Geometry check sheet. Reference: the model listing, model coordinates, mm. Give positions to 0.01 mm unless a question says otherwise; leave off trailing zeros. Loops run counter-clockwise (first coordinate to the right, second up) from the corner with the lowest first, then second, coordinate; pieces in that order, holes last. Notation, with made-up numbers: (85, 27.5) -> (132, 27.5) arc R19 cw to (132, 46.5) -> close; hole circle Ø2 at (48, 84.5). An arc over 180 degrees is marked (long way). One line per item, written item: value. Start each with the question number.
(1) Scan lines: line 1 along Y through (x, z) = (19, 1.2) (3 decimals); line 2 along Y through (x, z) = (-104.5, 1.9) (3 decimals); line 3 along Y through (x, z) = (24, 0.5) (3 decimals). Record each from-to range of solid material in increasing order. Write a range as from..to.
(2) Sectioned sample at C-C, the plane z = 0.55. State how many separate pieces and enclosed holes the cut face has, then the cut area to 3 significant figures.
(3) Sectioned sample at A-A, the plane x = 95.25. Record the cut outline in (y, z) (3 decimals).
(4) Draft check along X on faces 1 (the face through (-2, -3, 0)), 2 (the face through (103.9, 0.95, 1.57)). Enter one of: pulls with the +X half, pulls with the -X half, needs draft (parallel to the pull), parting line crosses it, or undercut.
(5) Sectioned sample at B-B, the plane x = -76.2. Record the cut outline in (y, z) (3 decimals).
Autodesk Inventor part; units mm, degrees
ref_plane "YZ Plane" through (0, 0, 0) normal (1, 0, 0) x (0, 1, 0)
ref_plane "XZ Plane" through (0, 0, 0) normal (0, 1, 0) x (-1, 0, 0)
ref_plane "XY Plane" through (0, 0, 0) normal (0, 0, 1) x (1, 0, 0)
sketch "Sketch1" plane through (0, 0, 0) normal (0, 0, 1) x (1, 0, 0)
  line L0 (-114.3, -15.875) -> (114.3, -15.875)
  line L1 (114.3, -15.875) -> (114.3, 15.875)
  line L2 (114.3, 15.875) -> (-114.3, 15.875)
  line L3 (-114.3, 15.875) -> (-114.3, -15.875)
  line L4 (-114.3, -15.875) -> (114.3, 15.875) construction
  line L5 (114.3, -15.875) -> (-114.3, 15.875) construction
  line L6 (-107.95, 9.525) -> (-82.55, 9.525) construction
  line L7 (-107.95, 6.9596) -> (-82.55, 6.9596)
  line L8 (-82.55, 12.0904) -> (-107.95, 12.0904)
  arc A0 (-107.95, 12.0904) -> (-107.95, 6.9596) centre (-107.95, 9.525) ccw
  arc A1 (-82.55, 6.9596) -> (-82.55, 12.0904) centre (-82.55, 9.525) ccw
  line L9 (-69.85, 9.525) -> (-44.45, 9.525) construction
  line L10 (-69.85, 6.9596) -> (-44.45, 6.9596)
  line L11 (-44.45, 12.0904) -> (-69.85, 12.0904)
  arc A2 (-69.85, 12.0904) -> (-69.85, 6.9596) centre (-69.85, 9.525) ccw
  arc A3 (-44.45, 6.9596) -> (-44.45, 12.0904) centre (-44.45, 9.525) ccw
  line L12 (-31.75, 9.525) -> (-6.35, 9.525) construction
  line L13 (-31.75, 6.9596) -> (-6.35, 6.9596)
  line L14 (-6.35, 12.0904) -> (-31.75, 12.0904)
  arc A4 (-31.75, 12.0904) -> (-31.75, 6.9596) centre (-31.75, 9.525) ccw
  arc A5 (-6.35, 6.9596) -> (-6.35, 12.0904) centre (-6.35, 9.525) ccw
  line L15 (6.35, 9.525) -> (31.75, 9.525) construction
  line L16 (6.35, 6.9596) -> (31.75, 6.9596)
  line L17 (31.75, 12.0904) -> (6.35, 12.0904)
  arc A6 (6.35, 12.0904) -> (6.35, 6.9596) centre (6.35, 9.525) ccw
  arc A7 (31.75, 6.9596) -> (31.75, 12.0904) centre (31.75, 9.525) ccw
  line L18 (44.45, 9.525) -> (69.85, 9.525) construction
  line L19 (44.45, 6.9596) -> (69.85, 6.9596)
  line L20 (69.85, 12.0904) -> (44.45, 12.0904)
  arc A8 (44.45, 12.0904) -> (44.45, 6.9596) centre (44.45, 9.525) ccw
  arc A9 (69.85, 6.9596) -> (69.85, 12.0904) centre (69.85, 9.525) ccw
  line L21 (82.55, 9.525) -> (107.95, 9.525) construction
  line L22 (82.55, 6.9596) -> (107.95, 6.9596)
  line L23 (107.95, 12.0904) -> (82.55, 12.0904)
  arc A10 (82.55, 12.0904) -> (82.55, 6.9596) centre (82.55, 9.525) ccw
  arc A11 (107.95, 6.9596) -> (107.95, 12.0904) centre (107.95, 9.525) ccw
  line L24 (-107.95, -9.525) -> (-82.55, -9.525) construction
  line L25 (-107.95, -12.0904) -> (-82.55, -12.0904)
  line L26 (-82.55, -6.9596) -> (-107.95, -6.9596)
  arc A12 (-107.95, -6.9596) -> (-107.95, -12.0904) centre (-107.95, -9.525) ccw
  arc A13 (-82.55, -12.0904) -> (-82.55, -6.9596) centre (-82.55, -9.525) ccw
  line L27 (-69.85, -9.525) -> (-44.45, -9.525) construction
  line L28 (-69.85, -12.0904) -> (-44.45, -12.0904)
  line L29 (-44.45, -6.9596) -> (-69.85, -6.9596)
  arc A14 (-69.85, -6.9596) -> (-69.85, -12.0904) centre (-69.85, -9.525) ccw
  arc A15 (-44.45, -12.0904) -> (-44.45, -6.9596) centre (-44.45, -9.525) ccw
  line L30 (-31.75, -9.525) -> (-6.35, -9.525) construction
  line L31 (-31.75, -12.0904) -> (-6.35, -12.0904)
  line L32 (-6.35, -6.9596) -> (-31.75, -6.9596)
  arc A16 (-31.75, -6.9596) -> (-31.75, -12.0904) centre (-31.75, -9.525) ccw
  arc A17 (-6.35, -12.0904) -> (-6.35, -6.9596) centre (-6.35, -9.525) ccw
  line L33 (6.35, -9.525) -> (31.75, -9.525) construction
  line L34 (6.35, -12.0904) -> (31.75, -12.0904)
  line L35 (31.75, -6.9596) -> (6.35, -6.9596)
  arc A18 (6.35, -6.9596) -> (6.35, -12.0904) centre (6.35, -9.525) ccw
  arc A19 (31.75, -12.0904) -> (31.75, -6.9596) centre (31.75, -9.525) ccw
  line L36 (44.45, -9.525) -> (69.85, -9.525) construction
  line L37 (44.45, -12.0904) -> (69.85, -12.0904)
  line L38 (69.85, -6.9596) -> (44.45, -6.9596)
  arc A20 (44.45, -6.9596) -> (44.45, -12.0904) centre (44.45, -9.525) ccw
  arc A21 (69.85, -12.0904) -> (69.85, -6.9596) centre (69.85, -9.525) ccw
  line L39 (82.55, -9.525) -> (107.95, -9.525) construction
  line L40 (82.55, -12.0904) -> (107.95, -12.0904)
  line L41 (107.95, -6.9596) -> (82.55, -6.9596)
  arc A22 (82.55, -6.9596) -> (82.55, -12.0904) centre (82.55, -9.525) ccw
  arc A23 (107.95, -12.0904) -> (107.95, -6.9596) centre (107.95, -9.525) ccw
  circle A24 centre (-107.95, 0) radius 2.4892
  circle A25 centre (-101.6, 0) radius 2.4892
  circle A26 centre (-95.25, 0) radius 2.4892
  circle A27 centre (-88.9, 0) radius 2.4892
  circle A28 centre (-82.55, 0) radius 2.4892
  circle A29 centre (-76.2, 0) radius 2.4892
  circle A30 centre (-69.85, 0) radius 2.4892
  circle A31 centre (-63.5, 0) radius 2.4892
  circle A32 centre (-57.15, 0) radius 2.4892
  circle A33 centre (-50.8, 0) radius 2.4892
  circle A34 centre (-44.45, 0) radius 2.4892
  circle A35 centre (-38.1, 0) radius 2.4892
  circle A36 centre (-31.75, 0) radius 2.4892
  circle A37 centre (-25.4, 0) radius 2.4892
  circle A38 centre (-19.05, 0) radius 2.4892
  circle A39 centre (-12.7, 0) radius 2.4892
  circle A40 centre (-6.35, 0) radius 2.4892
  circle A41 centre (0, 0) radius 2.4892
  circle A42 centre (6.35, 0) radius 2.4892
  circle A43 centre (12.7, 0) radius 2.4892
  circle A44 centre (19.05, 0) radius 2.4892
  circle A45 centre (25.4, 0) radius 2.4892
  circle A46 centre (31.75, 0) radius 2.4892
  circle A47 centre (38.1, 0) radius 2.4892
  circle A48 centre (44.45, 0) radius 2.4892
  circle A49 centre (50.8, 0) radius 2.4892
  circle A50 centre (57.15, 0) radius 2.4892
  circle A51 centre (63.5, 0) radius 2.4892
  circle A52 centre (69.85, 0) radius 2.4892
  circle A53 centre (76.2, 0) radius 2.4892
  circle A54 centre (82.55, 0) radius 2.4892
  circle A55 centre (88.9, 0) radius 2.4892
  circle A56 centre (95.25, 0) radius 2.4892
  circle A57 centre (101.6, 0) radius 2.4892
  circle A58 centre (107.95, 0) radius 2.4892
  point P0 (0, 0)
  point P1 (-95.25, 9.525)
  point P2 (-57.15, 9.525)
  point P3 (-19.05, 9.525)
  point P4 (19.05, 9.525)
  point P5 (57.15, 9.525)
  point P6 (95.25, 9.525)
  point P7 (-95.25, -9.525)
  point P8 (-57.15, -9.525)
  point P9 (-19.05, -9.525)
  point P10 (19.05, -9.525)
  point P11 (57.15, -9.525)
  point P12 (95.25, -9.525)
  dimension "d0" = 228.6
  dimension "d1" = 31.75
  dimension "d2" = 2.5654
  dimension "d3" = 25.4
  dimension "d4" = 6.35
  dimension "d5" = 6.35
  dimension "d8" = 38.1
  dimension "d11" = 19.05
  dimension "d14" = 6.35
  dimension "d17" = 6.35
  dimension "d22" = 4.9784
extrude "Extrusion1" add sketch "Sketch1" along normal blind 3.175
properties part number "QuickPrototypeplateB"
Calculated:
1. line 1: y = -15.875..-12.09, -6.96..-2.489, 2.489..6.96, 12.09..15.875
1. line 2: y = -15.875..-12.09, -6.96..6.96, 12.09..15.875
1. line 3: y = -15.875..-12.09, -6.96..-2.058, 2.058..6.96, 12.09..15.875
2. separate pieces: 1
2. enclosed holes: 47
2. area: 4,760 mm2
3. outline: (-15.875, 0) -> (-12.09, 0) -> (-12.09, 3.175) -> (-15.875, 3.175) -> close; (-6.96, 0) -> (-2.489, 0) -> (-2.489, 3.175) -> (-6.96, 3.175) -> close; (2.489, 0) -> (6.96, 0) -> (6.96, 3.175) -> (2.489, 3.175) -> close; (12.09, 0) -> (15.875, 0) -> (15.875, 3.175) -> (12.09, 3.175) -> close
4. face 1: needs draft
4. face 2: undercut
5. outline: (-15.875, 0) -> (-2.489, 0) -> (-2.489, 3.175) -> (-15.875, 3.175) -> close; (2.489, 0) -> (15.875, 0) -> (15.875, 3.175) -> (2.489, 3.175) -> close
